Build history of the part. All positions in model axes, mm. Give positions to 0.01 mm unless a question says otherwise; leave off trailing zeros. Order: outer loops, then holes, each group sorted by start corner. A loop starts at its lowest first (then second) coordinate and runs counter-clockwise, first axis right, second up. Notation, with made-up numbers: M 7.5,54.25 L 16.5,54.25 A15 cw 16.5,58.25 Z; hole C -38,79.25 d4. An arc over 180 degrees is marked long. Use CSV: the item, a comma, the result in double quotes. Start each with the question number.
Item 1: Pin check, flat tips, straight feed: P1, Ø1.5, axis at x = 27.5, z = 0, coming from the +Y side; P2, Ø1, axis at x = 4.5, z = 1, coming from the +Y side; P3, Ø0.9, axis at x = 27.5, z = 0, coming from the -Y side. Stop position of each tip, or through.
Item 2: Band-saw the part on A-A on x = 0. Write the cut outline in (y, z), plus the area to 3 significant figures.
Item 3: Band-saw the part on D-D on y = 48. Write the cut outline in (x, z), plus the area to 3 significant figures.
Item 4: Wall check: line 1 along X through (y, z) = (-1, 0.45); line 2 along Y through (x, z) = (0, -0.8); line 3 along Y through (x, z) = (-7, -0.7). Give the ranges that are in metal, low to high.
Item 5: Band-saw the part on C-C on z = 1.05. Give the number of separate pieces and of enclosed holes in the cut face, plus the area to 3 significant figures.
Item 6: Band-saw the part on B-B on x = -45. Write the cut outline in (y, z).
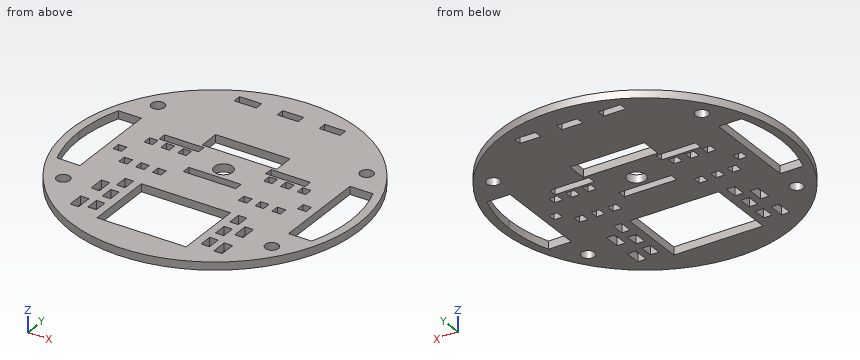
from build123d import *

# Parameters (mm, degrees)
F0_R     = 55
F0_R_2   = 2.5
F0_W     = 3.2
F0_H     = 6.1
F0_H_2   = 5
F0_H_3   = 3.2
F0_W_2   = 15
F0_W_3   = 8.41237
F0_W_4   = 8
F0_R_3   = 3.5
F1_DEPTH = 1.5


with BuildPart() as f1:
    # F0 (on Top) → F1 (new body, symmetric)
    with BuildSketch(Plane.XY):
        Circle(F0_R)
        with Locations((-39.8, -27.75)):
            Circle(F0_R_2, mode=Mode.SUBTRACT)
        with Locations((-27.4, -37.25)):
            Rectangle(F0_W, F0_H, mode=Mode.SUBTRACT)
        with Locations((-21.6, -36.3)):
            Rectangle(F0_W, F0_H_2, mode=Mode.SUBTRACT)
        with Locations((-21.6, -27.9)):
            Rectangle(F0_W, F0_H_2, mode=Mode.SUBTRACT)
        with Locations((-29.2, -7.4)):
            Rectangle(F0_W, F0_H_3, mode=Mode.SUBTRACT)
        with Locations((-35.2, -1.6)):
            Rectangle(F0_W, F0_H_3, mode=Mode.SUBTRACT)
        with Locations((-27.4, -25.05)):
            Rectangle(F0_W, F0_H, mode=Mode.SUBTRACT)
        with Locations((-21.6, -19.5)):
            Rectangle(F0_W, F0_H_2, mode=Mode.SUBTRACT)
        with Locations((-22.8, -7.4)):
            Rectangle(F0_W, F0_H_3, mode=Mode.SUBTRACT)
        with Locations((-16.4, -7.4)):
            Rectangle(F0_W, F0_H_3, mode=Mode.SUBTRACT)
        Polygon((-17, -17), (0, -17), (17, -17), (17, -43), (-17, -43), align=None, mode=Mode.SUBTRACT)
        with Locations((21.6, -36.3)):
            Rectangle(F0_W, F0_H_2, mode=Mode.SUBTRACT)
        with Locations((27.4, -37.25)):
            Rectangle(F0_W, F0_H, mode=Mode.SUBTRACT)
        with Locations((21.6, -27.9)):
            Rectangle(F0_W, F0_H_2, mode=Mode.SUBTRACT)
        with Locations((39.8, -27.75)):
            Circle(F0_R_2, mode=Mode.SUBTRACT)
        with Locations((27.4, -25.05)):
            Rectangle(F0_W, F0_H, mode=Mode.SUBTRACT)
        with Locations((21.6, -19.5)):
            Rectangle(F0_W, F0_H_2, mode=Mode.SUBTRACT)
        Polygon((-10, 0), (0, 0), (10, 0), (10, -3.2), (-10, -3.2), align=None, mode=Mode.SUBTRACT)
        with Locations((16.4, -7.4)):
            Rectangle(F0_W, F0_H_3, mode=Mode.SUBTRACT)
        with Locations((22.8, -7.4)):
            Rectangle(F0_W, F0_H_3, mode=Mode.SUBTRACT)
        with Locations((29.2, -7.4)):
            Rectangle(F0_W, F0_H_3, mode=Mode.SUBTRACT)
        with Locations((35.2, -1.6)):
            Rectangle(F0_W, F0_H_3, mode=Mode.SUBTRACT)
        with BuildLine():
            Line((-44.8, 18), (-39.8, 18))
            Line((-39.8, 18), (-39.8, -18))
            Line((-39.8, -18), (-44.8, -18))
            Line((-44.8, -18), (-48.572008, -18))
            ThreePointArc((-48.572008, -18), (-50.986616, -9.143576), (-51.8, 0))
            ThreePointArc((-51.8, 0), (-50.986616, 9.143576), (-48.572008, 18))
            Line((-48.572008, 18), (-44.8, 18))
        make_face(mode=Mode.SUBTRACT)
        with Locations((-29.2, 7.4)):
            Rectangle(F0_W, F0_H_3, mode=Mode.SUBTRACT)
        with Locations((-22.8, 7.4)):
            Rectangle(F0_W, F0_H_3, mode=Mode.SUBTRACT)
        with Locations((-16.4, 7.4)):
            Rectangle(F0_W, F0_H_3, mode=Mode.SUBTRACT)
        with Locations((-20.3, 11.6)):
            Rectangle(F0_W_2, F0_H_3, mode=Mode.SUBTRACT)
        with Locations((-39.8, 27.75)):
            Circle(F0_R_2, mode=Mode.SUBTRACT)
        with Locations((-16.793815, 45.1)):
            Rectangle(F0_W_3, F0_H_3, mode=Mode.SUBTRACT)
        with Locations((-0.58763, 45.1)):
            Rectangle(F0_W_4, F0_H_3, mode=Mode.SUBTRACT)
        with Locations((0, 5)):
            Circle(F0_R_3, mode=Mode.SUBTRACT)
        with Locations((16.4, 7.4)):
            Rectangle(F0_W, F0_H_3, mode=Mode.SUBTRACT)
        with Locations((20.3, 11.6)):
            Rectangle(F0_W_2, F0_H_3, mode=Mode.SUBTRACT)
        with Locations((22.8, 7.4)):
            Rectangle(F0_W, F0_H_3, mode=Mode.SUBTRACT)
        Polygon((-14.2, 22.2), (14.2, 22.2), (14.2, 15.2), (14.2, 14.3), (-14.2, 14.3), (-14.2, 15.2), align=None, mode=Mode.SUBTRACT)
        with Locations((29.2, 7.4)):
            Rectangle(F0_W, F0_H_3, mode=Mode.SUBTRACT)
        with BuildLine():
            Line((48.572008, -18), (44.8, -18))
            Line((44.8, -18), (39.8, -18))
            Line((39.8, -18), (39.8, 18))
            Line((39.8, 18), (44.8, 18))
            Line((44.8, 18), (48.572008, 18))
            ThreePointArc((48.572008, 18), (50.986616, 9.143576), (51.8, 0))
            ThreePointArc((51.8, 0), (50.986616, -9.143576), (48.572008, -18))
        make_face(mode=Mode.SUBTRACT)
        with Locations((15.41237, 45.1)):
            Rectangle(F0_W_4, F0_H_3, mode=Mode.SUBTRACT)
        with Locations((39.8, 27.75)):
            Circle(F0_R_2, mode=Mode.SUBTRACT)
    extrude(amount=F1_DEPTH, both=True)


solid = f1.part
Model answer:
1,P1,"stops at y = 48.06"
1,P2,"stops at y = 54.85"
1,P3,"stops at y = -47.89"
2,outline,"M -55,-1.5 L -43,-1.5 L -43,1.5 L -55,1.5 Z; M -17,-1.5 L -3.2,-1.5 L -3.2,1.5 L -17,1.5 Z; M 0,-1.5 L 1.5,-1.5 L 1.5,1.5 L 0,1.5 Z; M 8.5,-1.5 L 14.3,-1.5 L 14.3,1.5 L 8.5,1.5 Z; M 22.2,-1.5 L 43.5,-1.5 L 43.5,1.5 L 22.2,1.5 Z; M 46.7,-1.5 L 55,-1.5 L 55,1.5 L 46.7,1.5 Z"
2,area,"188 mm^2"
3,outline,"M -26.85,-1.5 L 26.85,-1.5 L 26.85,1.5 L -26.85,1.5 Z"
3,area,"161 mm^2"
4,line 1,"x = -54.99 to -51.79, -39.8 to -36.8, -33.6 to -10, 10 to 33.6, 36.8 to 39.8, 51.79 to 54.99"
4,line 2,"y = -55 to -43, -17 to -3.2, 0 to 1.5, 8.5 to 14.3, 22.2 to 43.5, 46.7 to 55"
4,line 3,"y = -54.55 to -43, -17 to -3.2, 0 to 14.3, 22.2 to 54.55"
5,separate pieces,"1"
5,enclosed holes,"39"
5,area,"6,930 mm^2"
6,outline,"M -31.62,-1.5 L -18,-1.5 L -18,1.5 L -31.62,1.5 Z; M 18,-1.5 L 31.62,-1.5 L 31.62,1.5 L 18,1.5 Z"
